Build history of the part. All positions in model axes, mm. Face numbers are marked on the shaded views. A direction names the side the tool comes from. Give positions to 0.01 mm unless a question says otherwise; leave off trailing zeros. Order: outer loops, then holes, each group sorted by start corner. A loop starts at its lowest first (then second) coordinate and runs counter-clockwise, first axis right, second up. Notation, with made-up numbers: (65, -32.75) - (95, -32.75) arc R17 ccw to (95, -6.75) - close; hole circle Ø8 at (-23, 67.25). An arc over 180 degrees is marked (long way). Write each question's results on one line, items separated by ' | '. Start each with the question number.
1) Cut at D-D on x = -4.5. List the corners of the cut face in (y, z), plus the area to 3 significant figures.
2) Drop flat-ended pins along their axis: pin 1 Ø2.5 at (x, z) = (5.45, 0) entering from -Y; pin 2 Ø1.5 at (y, z) = (-3.5, 6) entering from +X. Give the stop position or say it passes through.
3) Cut at A-A on z = 0. List the corners of the cut face in (x, y), plus the area to 3 significant figures.
4) Cut at B-B on x = 0. List the corners of the cut face in (y, z).
5) Cut at C-C on y = -2.7. List the corners of the cut face in (x, z), plus the area to 3 significant figures.
6) Tool access for the marked faces 4 and 5: list every direction of +Z, -Z, +X, -X, +Y, -Y with a clear straight run to the whole face (end or side of a thin tool).
7) Drill centre lines: line 1 along X through (y, z) = (-3.65, 0); line 2 along X through (y, z) = (-3.55, 1.25); line 3 along X through (y, z) = (-1.25, -1.75). Where is each one in solid material? Low to high. Write a range as from..to.
8) Two-plate mould, pull along Z, no slides. Class the marked faces 1, 2 and 3: +Z half, -Z half, draft (parallel to the pull), parting line (faces both ways), or undercut.
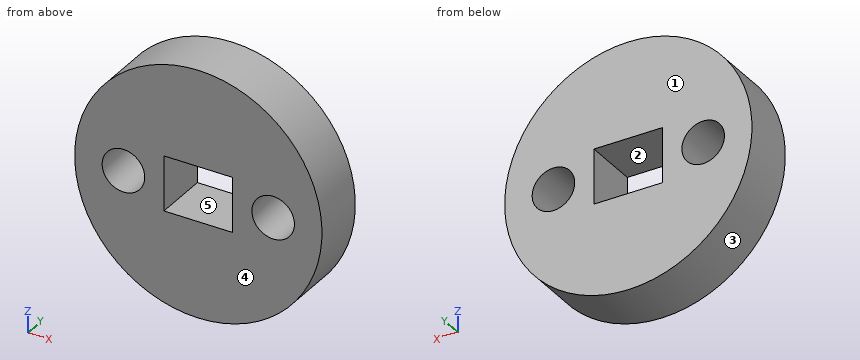
from build123d import *

# Parameters (mm, degrees)
SKETCH1_R          = 9
BASE_FLANGE1_DEPTH = 4
SKETCH7_R          = 1.55
CUT_EXTRUDE2_DEPTH = 10
SKETCH8_W          = 5
SKETCH8_H          = 4
CUT_EXTRUDE3_DEPTH = 10


# Sheet-metal steps are written as plain solids
with BuildPart() as part:
    # Sketch1 → Base-Flange1 (new body)
    with BuildSketch(Plane(origin=(0, 0, 0), x_dir=(1, 0, 0), z_dir=(0, 1, 0))):
        with Locations(Location((0, 0, 0), (0, 0, 270))):
            Circle(SKETCH1_R)
    extrude(amount=-BASE_FLANGE1_DEPTH)

    # Sketch7 → Cut-Extrude2 (cut)
    with BuildSketch(Plane(origin=(0, 0, 0), x_dir=(1, 0, 0), z_dir=(0, 1, 0))):
        with Locations(Location((-5.45, 0, 0), (0, 0, 270))):
            Circle(SKETCH7_R)
        with Locations(Location((5.45, 0, 0), (0, 0, 270))):
            Circle(SKETCH7_R)
    extrude(amount=-CUT_EXTRUDE2_DEPTH, mode=Mode.SUBTRACT)

    # Sketch8 → Cut-Extrude3 (cut)
    with BuildSketch(Plane(origin=(0, 0, 0), x_dir=(1, 0, 0), z_dir=(0, 1, 0))):
        Rectangle(SKETCH8_W, SKETCH8_H)
    extrude(amount=-CUT_EXTRUDE3_DEPTH, mode=Mode.SUBTRACT)


solid = part.part
Results:
1) outline: (-4, -7.79) - (0, -7.79) - (0, -1.22) - (-4, -1.22) - close; (-4, 1.22) - (0, 1.22) - (0, 7.79) - (-4, 7.79) - close | area: 52.6 mm^2
2) pin 1: through | pin 2: x = 7.31
3) outline: (-9, -4) - (-7, -4) - (-7, 0) - (-9, 0) - close; (-3.9, -4) - (-2.5, -4) - (-2.5, 0) - (-3.9, 0) - close; (2.5, -4) - (3.9, -4) - (3.9, 0) - (2.5, 0) - close; (7, -4) - (9, -4) - (9, 0) - (7, 0) - close | area: 27.2 mm^2
4) outline: (-4, -9) - (0, -9) - (0, -2) - (-4, -2) - close; (-4, 2) - (0, 2) - (0, 9) - (-4, 9) - close
5) outline: circle Ø18 at (0, 0); hole circle Ø3.1 at (-5.45, 0); hole (-2.5, -2) - (2.5, -2) - (2.5, 2) - (-2.5, 2) - close; hole circle Ø3.1 at (5.45, 0) | area: 219 mm^2
6) face 4: +Z, -Z, +X, -X, -Y | face 5: +Y, -Y
7) line 1: -9..-7, -3.9..-2.5, 2.5..3.9, 7..9 | line 2: -8.91..-6.37, -4.53..-2.5, 2.5..4.53, 6.37..8.91 | line 3: -8.83..-2.5, 2.5..8.83
8) face 1: draft | face 2: undercut | face 3: parting line
